Input: part model. Units: mm. Frame: model coordinates. Face numbers are marked on the shaded views. A direction names the side the tool comes from. Give positions to 0.01 mm unless a question says otherwise; leave off trailing zeros. Loops run counter-clockwise (first coordinate to the right, second up) from the corner with the lowest first, then second, coordinate; pieces in that order, holes last. Notation, with made-up numbers: (88, 81.25) -> (99, 81.25) arc R28 cw to (99, 110.25) -> close; hole circle Ø5 at (20, 11). An arc over 180 degrees is marked (long way). Answer as a JSON object with one key per item and string values.
```python
from build123d import *

# Parameters (mm, degrees)
F0_W      = 30
F0_H      = 50
F1_DEPTH  = 15
F2_W      = 30
F2_H      = 30
F3_DEPTH  = 150
F4_DEPTH  = 160
F6_DEPTH  = 30
F7_W      = 16.00820072
F7_H      = 6
F8_DEPTH  = 30
F9_DEPTH  = 15
F10_DEPTH = 5


with BuildPart() as f1:
    # F0 (on Top) → F1 (new body)
    with BuildSketch(Plane.XY):
        Rectangle(F0_W, F0_H)
    extrude(amount=F1_DEPTH)

    # F2 (on face) → F3 (join)
    with BuildSketch(Plane.XY.offset(15)):
        Rectangle(F2_W, F2_H)
    extrude(amount=F3_DEPTH)

    # F4 (add): a face of the model
    f4_faces = [f1.faces().sort_by_distance(p)[0] for p in [
        (0, -25, 7.5),
    ]]
    extrude(f4_faces, amount=F4_DEPTH)

    # F5 (on face) → F6 (join)
    with BuildSketch(Plane(origin=(-15, 0, 0), x_dir=(0, -1, 0), z_dir=(-1, 0, 0))):
        Polygon((144.7644245625, 15), (174.7644245625, 15), (15, 165), (15, 135), align=None)
    extrude(amount=-F6_DEPTH)

    # F7 (on face) → F8 (join)
    with BuildSketch(Plane(origin=(-15, 0, 0), x_dir=(0, -1, 0), z_dir=(-1, 0, 0))):
        Polygon((-15, 189), (-15, 165), (15, 165), (15, 195), (-15, 195), align=None)
        with Locations((-23.00410036, 192)):
            Rectangle(F7_W, F7_H)
    extrude(amount=-F8_DEPTH)

    # F9 (add): a face of the model
    f9_faces = [f1.faces().sort_by_distance(p)[0] for p in [
        (0, 25, 7.5),
    ]]
    extrude(f9_faces, amount=F9_DEPTH)

    # F10 (add): a face of the model
    f10_faces = [f1.faces().sort_by_distance(p)[0] for p in [
        (0, 23.00410036, 189),
    ]]
    extrude(f10_faces, amount=F10_DEPTH)


solid = f1.part
```
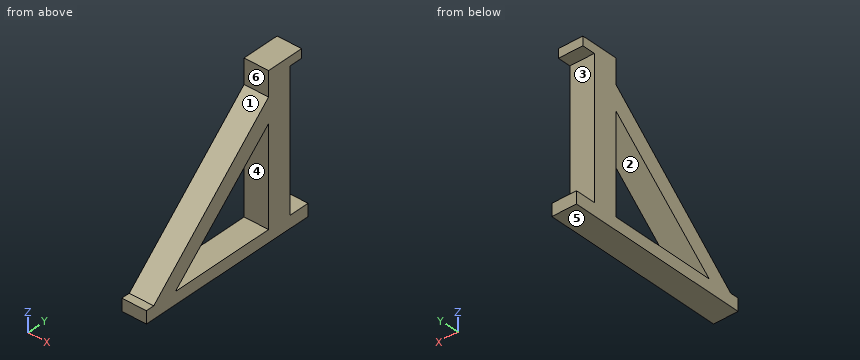
Q1. Section C-C, the plane z = 112. Return the cut outline in (x, y).
Evaluation:
{"outline": "(-15, -71.45) -> (15, -71.45) -> (15, -39.87) -> (-15, -39.87) -> close; (-15, -15) -> (15, -15) -> (15, 15) -> (-15, 15) -> close"}
Q2. Pin query (flat end, axial travel): pin 1 (15 mm diameter, centred on x = 7, y = -49.5, fed in from +Z); pin 2 (6 mm diameter, centred on x = -1.5, z = 26.5, fed in from +Y); pin 3 (5.5 mm diameter, centred on x = -3.5, z = 187, fed in from +Y). Return the tip coordinate at first contact, or that it passes through.
Evaluation:
{"pin 1": "stops at z = 139.65", "pin 2": "stops at y = 15", "pin 3": "stops at y = 31.01"}
Q3. Access query for the marked faces 1, 2 and 3. Directions: +Z, -Z, +X, -X, +Y, -Y. A direction counts if a zero-diameter tool reaches every point of the face in a straight line with its end or side. Return the directions, or none.
Evaluation:
{"face 1": "+Z, +X, -X, -Y", "face 2": "+X, -X", "face 3": "+X, -X, +Y"}
Q4. Draft query along Z for the marked faces 4, 5 and 6. Return one class per face: +Z half, -Z half, draft (parallel to the pull), parting line (faces both ways), or undercut.
Evaluation:
{"face 4": "undercut", "face 5": "-Z half", "face 6": "draft"}
Q5. Section B-B, the plane x = -4. Return the cut outline in (y, z).
Evaluation:
{"outline": "(-185, 0) -> (40, 0) -> (40, 15) -> (15, 15) -> (15, 184) -> (31.01, 184) -> (31.01, 195) -> (-15, 195) -> (-15, 165) -> (-174.76, 15) -> (-185, 15) -> close; hole (-144.76, 15) -> (-15, 15) -> (-15, 135) -> close"}
Q6. Section A-A, the plane y = 24. Return the cut outline in (x, z), then the cut area to 3 significant figures.
Evaluation:
{"outline": "(-15, 0) -> (15, 0) -> (15, 15) -> (-15, 15) -> close; (-15, 184) -> (15, 184) -> (15, 195) -> (-15, 195) -> close", "area": "780 mm2"}
Q7. Ray query, line 1 along Y through (x, z) = (-2.5, 171); line 2 along Z through (x, y) = (-12, 21.5); line 3 along Y through (x, z) = (6, 120). Return the intervals inside material, ascending.
Evaluation:
{"line 1": "y = -15 to 15", "line 2": "z = 0 to 15, 184 to 195", "line 3": "y = -62.93 to -31.22, -15 to 15"}
Q8. Section D-D, the plane z = 148. Return the cut outline in (x, y), then the cut area to 3 significant figures.
Evaluation:
{"outline": "(-15, -33.11) -> (15, -33.11) -> (15, 15) -> (-15, 15) -> close", "area": "1,440 mm2"}
